Design review of the part built by this model. Coordinates are the model's own, in mm. A direction names the side the tool comes from. Round coordinates to 2 decimals unless told otherwise and drop trailing zeros. Loops run counter-clockwise (first coordinate to the right, second up) from the corner with the lowest first, then second, coordinate; pieces in that order, holes last. Notation, with made-up numbers: (68.5, 18) - (107.5, 18) arc R26 cw to (107.5, 38) - close; hole circle Ø8 at (84.25, 29.5). An arc over 180 degrees is marked (long way). Use one line per item in the form item = value. Start each with the question number.
(1) The part is to be moulded in two halves that separate along Z. For faces 1 (the flat face through (126, -4, -1)), 2 (the cylindrical face through (95.87, -9.49, 6.17)), 3 (the flat face through (-1, -4, -21)), say which applies: released by +Z, released by -Z, zero draft, split by the parting line, or undercut.
(2) For pin 1 (0.8 mm diameter, centred on y = -9.5, z = -18.5, fed in from +X); pin 2 (4 mm diameter, centred on y = -7, z = 10.5, fed in from -X); pin 3 (0.8 mm diameter, centred on x = -7.5, y = -9.5, fed in from +Z) (3 decimals); pin 4 (23 mm diameter, centred on x = 75, z = 0, fed in from +Y), all flat-tipped, find the tip position at first contact; note any pin that passes through.
(3) We need section B-B, the plane x = 0. Write out the cut boundary in (y, z), then the cut area to 3 significant figures.
(4) We need section A-A, the plane y = -3.25. Write out the cut boundary in (x, z), then the cut area to 3 significant figures.
(5) Wall thickness on probe 1 along X at (y, z) = (-4, 0.5); probe 2 along X at (y, z) = (-6.75, 1); probe 3 along Z at (x, y) = (0, -5.25): over which ranges is each line inside the solid? List them lowest first. Write a range as [from, to].
(6) Machinability: for faces 4 (the flat face through (-69, -4, -23)), 5 (the cylindrical face through (92.42, -9.49, -7.96)), 6 (the flat face through (-126, -4, -1)), 7 (the flat face through (1, -4, 21)), which of the approach directions +Z, -Z, +X, -X, +Y, -Y give a long, thin tool a straight path to every point of the face, cutting with its end or side? Answer none if there is none.
(7) We need section C-C, the plane x = -30.5. Write out the cut boundary in (y, z).
from build123d import *

# Parameters (mm, degrees)
F0_R     = 10
F0_R_2   = 6.5
F1_DEPTH = 10
F2_DEPTH = 9
F3_R     = 1


with BuildPart() as f1:
    # F0 (on Front) → F1 (new body)
    with BuildSketch(Plane.XZ):
        with BuildLine():
            Line((69, -25), (77.6, -25))
            ThreePointArc((77.6, -25), (99.482843, -9.173343), (126, -4.05648))
            Line((126, -4.05648), (126, 2.04352))
            ThreePointArc((126, 2.04352), (99.215863, 8.073528), (77.6, 25))
            Line((77.6, 25), (69, 25))
            Line((69, 25), (69, 21))
            Line((69, 21), (-69, 21))
            Line((-69, 21), (-69, 25))
            Line((-69, 25), (-77.6, 25))
            ThreePointArc((-77.6, 25), (-99.215863, 8.073528), (-126, 2.04352))
            Line((-126, 2.04352), (-126, -4.05648))
            ThreePointArc((-126, -4.05648), (-99.482843, -9.173343), (-77.6, -25))
            Line((-77.6, -25), (-69, -25))
            Line((-69, -25), (-69, -21))
            Line((-69, -21), (69, -21))
            Line((69, -21), (69, -25))
        make_face()
        with BuildLine():
            Line((-76.109897, 21.81), (-72.19, 21.81))
            Line((-72.19, 21.81), (-72.19, 17.81))
            Line((-72.19, 17.81), (72.19, 17.81))
            Line((72.19, 17.81), (72.19, 21.81))
            Line((72.19, 21.81), (76.109897, 21.81))
            ThreePointArc((76.109897, 21.81), (96.187204, 6.008289), (120.774538, -0.938314))
            ThreePointArc((120.774538, -0.938314), (96.452782, -7.039668), (76.189226, -21.81))
            Line((76.189226, -21.81), (72.19, -21.81))
            Line((72.19, -21.81), (72.19, -17.81))
            Line((72.19, -17.81), (-72.19, -17.81))
            Line((-72.19, -17.81), (-72.19, -21.81))
            Line((-72.19, -21.81), (-76.189226, -21.81))
            ThreePointArc((-76.189226, -21.81), (-96.452782, -7.039668), (-120.774538, -0.938314))
            ThreePointArc((-120.774538, -0.938314), (-96.187204, 6.008289), (-76.109897, 21.81))
        make_face(mode=Mode.SUBTRACT)
        with BuildLine():
            Line((-73.19, 16.81), (-73.19, 20.81))
            Line((-73.19, 20.81), (-75.651859, 20.81))
            ThreePointArc((-75.651859, 20.81), (-92.453393, 6.905154), (-112.842512, -0.835655))
            ThreePointArc((-112.842512, -0.835655), (-92.625004, -7.802454), (-75.651859, -20.81))
            Line((-75.651859, -20.81), (-73.19, -20.81))
            Line((-73.19, -20.81), (-73.19, -16.81))
            Line((-73.19, -16.81), (73.19, -16.81))
            Line((73.19, -16.81), (73.19, -20.81))
            Line((73.19, -20.81), (75.755417, -20.81))
            ThreePointArc((75.755417, -20.81), (92.680477, -7.817723), (112.842512, -0.835655))
            ThreePointArc((112.842512, -0.835655), (92.453393, 6.905154), (75.651859, 20.81))
            Line((75.651859, 20.81), (73.19, 20.81))
            Line((73.19, 20.81), (73.19, 16.81))
            Line((73.19, 16.81), (-73.19, 16.81))
        make_face()
        with Locations((-75, 0)):
            Circle(F0_R, mode=Mode.SUBTRACT)
        Circle(F0_R_2, mode=Mode.SUBTRACT)
        with Locations((75, 0)):
            Circle(F0_R, mode=Mode.SUBTRACT)
    extrude(amount=F1_DEPTH)

    # F0 (on Front) → F2 (join)
    with BuildSketch(Plane.XZ):
        with BuildLine():
            Line((-72.19, 17.81), (-72.19, 21.81))
            Line((-72.19, 21.81), (-76.109897, 21.81))
            ThreePointArc((-76.109897, 21.81), (-96.187204, 6.008289), (-120.774538, -0.938314))
            ThreePointArc((-120.774538, -0.938314), (-96.452782, -7.039668), (-76.189226, -21.81))
            Line((-76.189226, -21.81), (-72.19, -21.81))
            Line((-72.19, -21.81), (-72.19, -17.81))
            Line((-72.19, -17.81), (72.19, -17.81))
            Line((72.19, -17.81), (72.19, -21.81))
            Line((72.19, -21.81), (76.189226, -21.81))
            ThreePointArc((76.189226, -21.81), (96.452782, -7.039668), (120.774538, -0.938314))
            ThreePointArc((120.774538, -0.938314), (96.187204, 6.008289), (76.109897, 21.81))
            Line((76.109897, 21.81), (72.19, 21.81))
            Line((72.19, 21.81), (72.19, 17.81))
            Line((72.19, 17.81), (-72.19, 17.81))
        make_face()
        with BuildLine():
            Line((-75.651859, 20.81), (-73.19, 20.81))
            Line((-73.19, 20.81), (-73.19, 16.81))
            Line((-73.19, 16.81), (73.19, 16.81))
            Line((73.19, 16.81), (73.19, 20.81))
            Line((73.19, 20.81), (75.651859, 20.81))
            ThreePointArc((75.651859, 20.81), (92.453393, 6.905154), (112.842512, -0.835655))
            ThreePointArc((112.842512, -0.835655), (92.680477, -7.817723), (75.755417, -20.81))
            Line((75.755417, -20.81), (73.19, -20.81))
            Line((73.19, -20.81), (73.19, -16.81))
            Line((73.19, -16.81), (-73.19, -16.81))
            Line((-73.19, -16.81), (-73.19, -20.81))
            Line((-73.19, -20.81), (-75.651859, -20.81))
            ThreePointArc((-75.651859, -20.81), (-92.625004, -7.802454), (-112.842512, -0.835655))
            ThreePointArc((-112.842512, -0.835655), (-92.453393, 6.905154), (-75.651859, 20.81))
        make_face(mode=Mode.SUBTRACT)
    extrude(amount=F2_DEPTH)

    # F3
    f3_edges = [f1.edges().sort_by_distance(p)[0] for p in [
        (-99.215863, -10, 8.073528),
        (-126, -10, -1.00648),
        (-99.482843, -10, -9.173343),
        (-73.3, -10, -25),
        (-69, -10, -23),
        (0, -10, -21),
        (-73.3, -10, 25),
        (-69, -10, 23),
        (0, -10, 21),
        (69, -10, -23),
        (73.3, -10, -25),
        (99.482843, -10, -9.173343),
        (126, -10, -1.00648),
        (99.215863, -10, 8.073528),
        (73.3, -10, 25),
        (69, -10, 23),
    ]]
    fillet(f3_edges, radius=F3_R)


solid = f1.part
Data:
q1.face_1 = zero draft
q1.face_2 = undercut
q1.face_3 = released by -Z
q2.pin_1 = 84.67
q2.pin_2 = -98.33
q2.pin_3 = 20.995
q2.pin_4 = 0
q3.outline = (-10, -20) arc R1 ccw to (-9, -21) - (0, -21) - (0, -6.5) - (-10, -6.5) - (-10, -16.81) - (-9, -16.81) - (-9, -17.81) - (-10, -17.81) - close; (-10, 6.5) - (0, 6.5) - (0, 21) - (-9, 21) arc R1 ccw to (-10, 20) - (-10, 17.81) - (-9, 17.81) - (-9, 16.81) - (-10, 16.81) - close
q3.area = 288 mm^2
q4.outline = (-126, -4.06) arc R62.5 cw to (-77.6, -25) - (-69, -25) - (-69, -21) - (69, -21) - (69, -25) - (77.6, -25) arc R62.5 cw to (126, -4.06) - (126, 2.04) arc R62.5 cw to (77.6, 25) - (69, 25) - (69, 21) - (-69, 21) - (-69, 25) - (-77.6, 25) arc R62.5 cw to (-126, 2.04) - close; hole circle Ø20 at (-75, 0); hole circle Ø13 at (0, 0); hole circle Ø20 at (75, 0)
q4.area = 7,760 mm^2
q5.probe_1 = [-126, -84.99], [-65.01, -6.48], [6.48, 65.01], [84.99, 126]
q5.probe_2 = [-126, -84.95], [-65.05, -6.42], [6.42, 65.05], [84.95, 126]
q5.probe_3 = [-21, -6.5], [6.5, 21]
q6.face_4 = -Z, +Y, -Y
q6.face_5 = -Y
q6.face_6 = +Z, -Z, -X, +Y, -Y
q6.face_7 = +Z, +Y, -Y
q7.outline = (-10, -20) arc R1 ccw to (-9, -21) - (0, -21) - (0, 21) - (-9, 21) arc R1 ccw to (-10, 20) - (-10, 17.81) - (-9, 17.81) - (-9, 16.81) - (-10, 16.81) - (-10, -16.81) - (-9, -16.81) - (-9, -17.81) - (-10, -17.81) - close
